CAD build for the part. Positions are in the model's coordinates, mm. Round coordinates to 2 decimals unless told otherwise and drop trailing zeros. Loops run counter-clockwise (first coordinate to the right, second up) from the corner with the lowest first, then second, coordinate; pieces in that order, holes last. Notation, with made-up numbers: (68, 54) - (96, 54) arc R22 ccw to (96, 82) - close; hole circle Ø2 at (43.5, -26.75). An arc over 180 degrees is marked (long way). Use one line per item in the form item = value.
from build123d import *

# Parameters (mm, degrees)
SKETCH1_W           = 35.5
SKETCH1_H           = 11.1
BOSS_EXTRUDE1_DEPTH = 5.75
FILLET1_R           = 1.5


with BuildPart() as part:
    # Sketch1 → Boss-Extrude1 (new body)
    with BuildSketch(Plane.XY):
        with Locations((17.75, 5.55)):
            Rectangle(SKETCH1_W, SKETCH1_H)
    extrude(amount=BOSS_EXTRUDE1_DEPTH)

    # Fillet1
    fillet1_edges = [part.edges().sort_by_distance(p)[0] for p in [
        (17.75, 11.1, 5.75),
        (0, 5.55, 5.75),
        (17.75, 11.1, 0),
        (17.75, 0, 0),
        (0, 5.55, 0),
        (17.75, 0, 5.75),
        (0, 11.1, 2.875),
        (0, 0, 2.875),
    ]]
    fillet(fillet1_edges, radius=FILLET1_R)


solid = part.part
1) Drill centre lines: probe 1 along X at (y, z) = (4.75, 4.35); probe 2 along X at (y, z) = (6, 5.5); probe 3 along Y at (x, z) = (18, 0.2). Where is each one in solid material? Low to high.
Report:
probe_1 = 0 to 35.5
probe_2 = 0.67 to 35.5
probe_3 = 0.75 to 10.35
2) Slice it at C-C (y = 1). Write the cut outline in (x, z).
Report:
outline = (0.09, 1.5) arc R1.41 ccw to (1.5, 0.09) - (35.5, 0.09) - (35.5, 5.66) - (1.5, 5.66) arc R1.41 ccw to (0.09, 4.25) - close
3) Slice it at B-B (z = 5.35). Write the cut outline in (x, y), plus the area to 3 significant figures.
Report:
outline = (0.48, 1.5) arc R1.02 ccw to (1.5, 0.48) - (35.5, 0.48) - (35.5, 10.62) - (1.5, 10.62) arc R1.02 ccw to (0.48, 9.6) - close
area = 355 mm^2
4) Slice it at A-A (x = 11). Write the cut outline in (y, z), plus the area to 3 significant figures.
Report:
outline = (0, 1.5) arc R1.5 ccw to (1.5, 0) - (9.6, 0) arc R1.5 ccw to (11.1, 1.5) - (11.1, 4.25) arc R1.5 ccw to (9.6, 5.75) - (1.5, 5.75) arc R1.5 ccw to (0, 4.25) - close
area = 61.9 mm^2
